The listing builds one solid part. Answer for the finished solid, in the listing's coordinates (mm). Face numbers are marked on the shaded views. A direction names the side the tool comes from. Coordinates: 2 decimals unless noted, no trailing zeros. Loops run counter-clockwise (first coordinate to the right, second up) from the corner with the lowest first, then second, coordinate; pieces in that order, holes last. Notation, with made-up numbers: M 78,69.5 L 115,69.5 A27 ccw 115,98.5 Z; hole C 47.5,66 d6. An arc over 180 degrees is marked long. Answer as a JSON object with one key per item and string values. Group by question number.
1. A cutting plane is placed at A-A on y = 16. Give the vertices of the cut face in (x, z), and give its area (3 significant figures).
2. Given pin 1 (13 mm diameter, centred on x = 3, z = -1.5, fed in from -Y); pin 2 (16 mm diameter, centred on x = 1.5, z = -2.5, fed in from -Y); pin 3 (3 mm diameter, centred on x = 0, y = 16, fed in from +Z); pin 4 (3 mm diameter, centred on x = 8, y = 17.5, fed in from +Z), each flat-ended and moving along its own axis, determine where each tip first touches the part or whether it passes through.
3. Determine the mould class of the marked faces 1, 2, 3 and 4 for opening direction X: released by +X, released by -X, zero draft, split by the parting line, or undercut.
4. A cutting plane is placed at B-B on x = -1. State how many separate pieces and enclosed holes the cut face has, and give its area (3 significant figures).
5. For the marked faces 5 and 6, determine the directions among +Z, -Z, +X, -X, +Y, -Y from which every point of the face is accessible in a straight line to the end or side of a thin tool.
6. Straight lines are drawn through the part: L1, parallel to Z at x = -0.5, y = 2; L2, parallel to Y at x = 14, z = -7; L3, parallel to Z at x = 0.5, y = 23.5. For each, find the intervals that lie inside material, in ascending order.
from build123d import *

# Parameters (mm, degrees)
CUT_EXTRUDE1_DEPTH      = 40.191835966
CUT_EXTRUDE1_DEPTH_BACK = 40.191835966
SKETCH3_R               = 2.5


with BuildPart() as part:
    # Sketch2 → Revolve1 (revolve)
    with BuildSketch(Plane.XY):
        with BuildLine():
            Line((16, 27), (14.5, 27))
            Line((14.5, 27), (14.5, 25.5))
            Line((14.5, 25.5), (16, 25.5))
            Line((16, 25.5), (16, 22.5))
            Line((16, 22.5), (14.5, 22.5))
            Line((14.5, 22.5), (14.5, 21))
            Line((14.5, 21), (16, 21))
            Line((16, 21), (16, 0))
            Line((16, 0), (13, 0))
            Line((13, 0), (13, 10))
            Line((13, 10), (10, 10))
            Line((10, 10), (10, 24))
            Line((10, 24), (0, 24))
            Line((0, 24), (0, 32))
            ThreePointArc((0, 32), (1.036981818, 31.899736945), (2.067335712, 31.745610948))
            Line((2.067335712, 31.745610948), (16, 29.288906321))
            Line((16, 29.288906321), (16, 27))
        make_face()
    revolve(axis=Axis((0, 0, 0), (0, 1, 0)))

    # Sketch3 → Cut-Extrude1 (cut, two sides: drawn at the far end of the back side and taken through both)
    with BuildSketch(Plane.XY.offset(-CUT_EXTRUDE1_DEPTH_BACK)):
        with Locations((0, 16)):
            Circle(SKETCH3_R)
    extrude(amount=CUT_EXTRUDE1_DEPTH + CUT_EXTRUDE1_DEPTH_BACK, mode=Mode.SUBTRACT)


solid = part.part
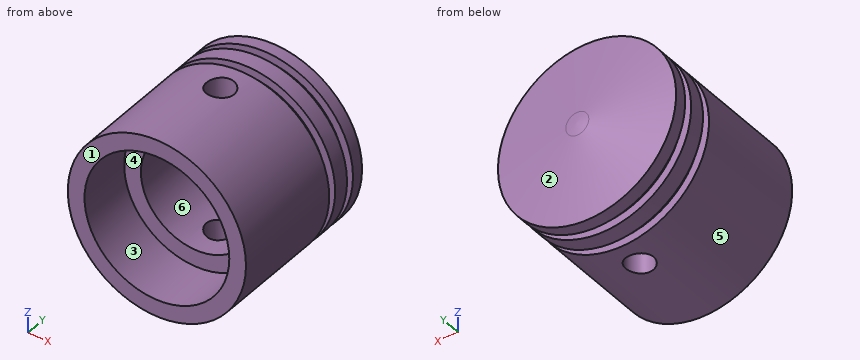
From the geometry:
{
 "1": {"outline": "M -2.5,-15.8 L -2.5,-9.68 A10 cw -2.5,9.68 L -2.5,15.8 A16 ccw Z; M 2.5,-15.8 A16 ccw 2.5,15.8 L 2.5,9.68 A10 cw 2.5,-9.68 Z", "area": "430 mm²"},
 "2": {"pin 1": "stops at y = 24", "pin 2": "stops at y = 10", "pin 3": "passes through", "pin 4": "stops at z = 14.62"},
 "3": {"face 1": "zero draft", "face 2": "split by the parting line", "face 3": "undercut", "face 4": "undercut"},
 "4": {"separate pieces": "3", "enclosed holes": "0", "area": "378 mm²"},
 "5": {"face 5": "+Y, -Y", "face 6": "-Y"},
 "6": {"L1": "z = -15.99 to -12.99, 12.99 to 15.99", "L2": "y = 0 to 21, 22.5 to 25.5, 27 to 29.35", "L3": "z = -15.99 to -9.99, 9.99 to 15.99"}
}
